Part print with two shaded views. Sizes in mm from the minimum x, y, z corner. Round coordinates to 2 decimals unless told otherwise and drop trailing zeros. Write each loop counter-clockwise with the first axis right and the second up, starting at its lowest first coordinate (ties: lowest second). Pieces come first, ordered by that corner, then holes. Notation, with made-up numbers: M 29,38.25 L 66,38.25 A37 ccw 66,74.25 Z; hole C 67.25,27.25 d2. An arc over 180 degrees is marked long. Use one line per item in the form item = value. Start each with the question number.
Item 1: Probe L1, parallel to X at y = 1.6, z = 12.7 (3 decimals); L2, parallel to Z at x = 12.7, y = 1.2 (3 decimals). List the from-to ranges inside material, lowest first.
Item 2: Flat gauge pins, fed straight in: pin 1 Ø5 at (x, z) = (88.9, 63.5) entering from -Y; pin 2 Ø1.3 at (y, z) = (1, 84) entering from -X. Where does each tip first touch, or does it go through?
Item 3: Cut at B-B, the plane z = 12.7. Give the cut face in (x, y) (3 decimals), then the cut area to 3 significant figures.
Item 4: Cut at D-D, the plane x = 12.7. Give the cut face in (y, z) (3 decimals).
Item 5: Cut at A-A, the plane x = 88.9. Give the cut face in (y, z) (3 decimals), then the cut area to 3 significant figures.
Item 6: Cut at C-C, the plane y = 1.1. Give the cut face in (x, z) (3 decimals), then the cut area to 3 significant figures.
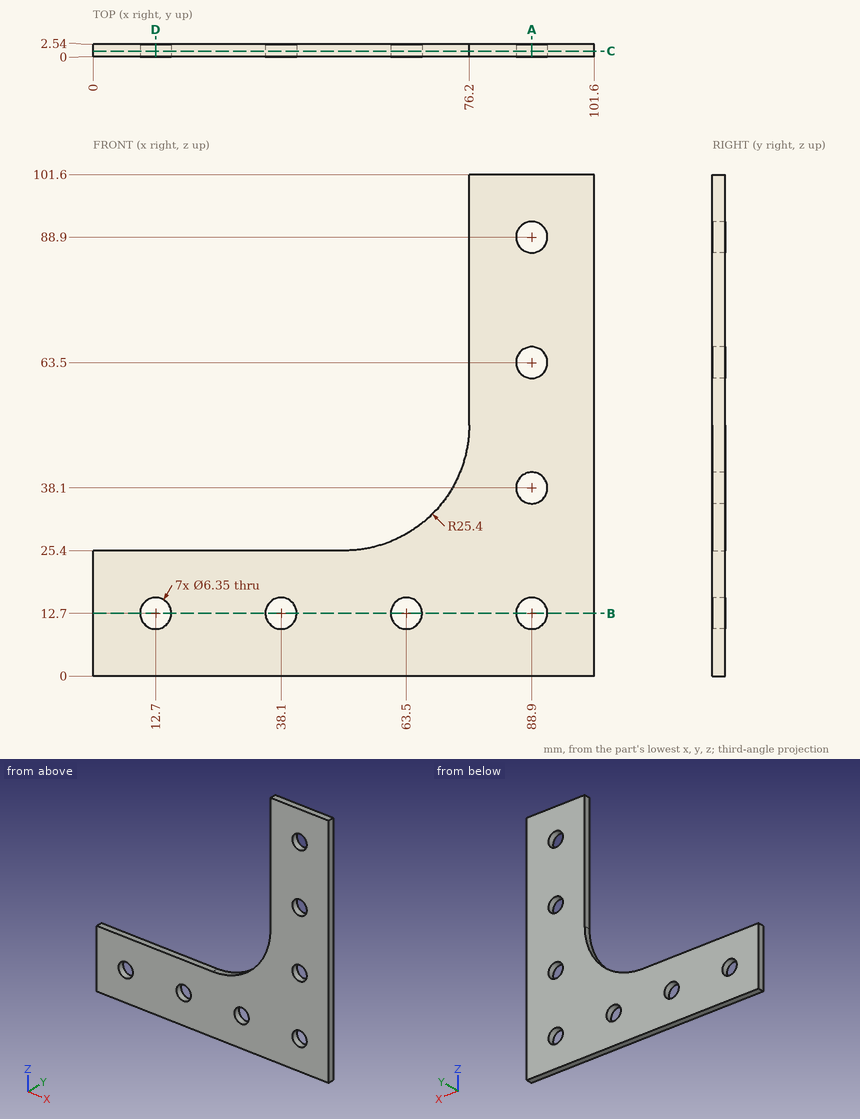
Model answer:
q1.L1 = 0 to 9.525, 15.875 to 34.925, 41.275 to 60.325, 66.675 to 85.725, 92.075 to 101.6
q1.L2 = 0 to 9.525, 15.875 to 25.4
q2.pin_1 = through
q2.pin_2 = 76.2
q3.outline = M 0,0 L 9.525,0 L 9.525,2.54 L 0,2.54 Z; M 15.875,0 L 34.925,0 L 34.925,2.54 L 15.875,2.54 Z; M 41.275,0 L 60.325,0 L 60.325,2.54 L 41.275,2.54 Z; M 66.675,0 L 85.725,0 L 85.725,2.54 L 66.675,2.54 Z; M 92.075,0 L 101.6,0 L 101.6,2.54 L 92.075,2.54 Z
q3.area = 194 mm²
q4.outline = M 0,0 L 2.54,0 L 2.54,9.525 L 0,9.525 Z; M 0,15.875 L 2.54,15.875 L 2.54,25.4 L 0,25.4 Z
q5.outline = M 0,0 L 2.54,0 L 2.54,9.525 L 0,9.525 Z; M 0,15.875 L 2.54,15.875 L 2.54,34.925 L 0,34.925 Z; M 0,41.275 L 2.54,41.275 L 2.54,60.325 L 0,60.325 Z; M 0,66.675 L 2.54,66.675 L 2.54,85.725 L 0,85.725 Z; M 0,92.075 L 2.54,92.075 L 2.54,101.6 L 0,101.6 Z
q5.area = 194 mm²
q6.outline = M 0,0 L 101.6,0 L 101.6,101.6 L 76.2,101.6 L 76.2,50.8 A25.4 cw 50.8,25.4 L 0,25.4 Z; hole C 12.7,12.7 d6.35; hole C 38.1,12.7 d6.35; hole C 63.5,12.7 d6.35; hole C 88.9,12.7 d6.35; hole C 88.9,38.1 d6.35; hole C 88.9,63.5 d6.35; hole C 88.9,88.9 d6.35
q6.area = 4,430 mm²
